CAD build for the part. Positions are in the model's coordinates, mm. A direction names the side the tool comes from. Round coordinates to 2 decimals unless told otherwise and drop trailing zeros. Write each loop counter-clockwise with the first axis right and the second up, starting at its lowest first coordinate (ties: lowest second). Pieces come first, ordered by that corner, then holes. Notation, with made-up numbers: (38.5, 65) - (77.5, 65) arc R23 cw to (77.5, 75) - close; hole circle Ø2 at (25, -0.75). An arc over 180 degrees is marked (long way). Answer in a Markdown table with one row per item.
```python
from build123d import *

# Parameters (mm, degrees)
BOSS_EXTRUDE1_DEPTH = 60
SKETCH4_W           = 10
SKETCH4_H           = 90
BOSS_EXTRUDE2_DEPTH = 45
SKETCH6_W           = 25
SKETCH6_H           = 10
BOSS_EXTRUDE3_DEPTH = 45
SKETCH8_W           = 10
SKETCH8_H           = 15
BOSS_EXTRUDE4_DEPTH = 90
CUT_EXTRUDE1_DEPTH  = 10
BOSS_EXTRUDE5_DEPTH = 20
CUT_EXTRUDE2_DEPTH  = 5
SKETCH12_W          = 10
SKETCH12_H          = 30.5
CUT_EXTRUDE3_DEPTH  = 5
BOSS_EXTRUDE6_DEPTH = 5


with BuildPart() as part:
    # Sketch1 → Boss-Extrude1 (new body)
    with BuildSketch(Plane(origin=(0, 0, 0), x_dir=(0, 0, -1), z_dir=(1, 0, 0))):
        Polygon((0, -10), (0, 90), (10, 90), (10, 0), (25, 0), (25, -10), align=None)
    extrude(amount=BOSS_EXTRUDE1_DEPTH)

    # Sketch4 → Boss-Extrude2 (add)
    with BuildSketch(Plane.ZY):
        with Locations((-5, 45)):
            Rectangle(SKETCH4_W, SKETCH4_H)
    extrude(amount=BOSS_EXTRUDE2_DEPTH)

    # Sketch6 → Boss-Extrude3 (add)
    with BuildSketch(Plane.ZY):
        with Locations((-12.5, -5)):
            Rectangle(SKETCH6_W, SKETCH6_H)
    extrude(amount=BOSS_EXTRUDE3_DEPTH)

    # Sketch8 → Boss-Extrude4 (add)
    with BuildSketch(Plane(origin=(0, 0, 0), x_dir=(1, 0, 0), z_dir=(0, 1, 0))):
        with Locations((-40, 17.5)):
            Rectangle(SKETCH8_W, SKETCH8_H)
    extrude(amount=BOSS_EXTRUDE4_DEPTH)

    # Sketch9 → Cut-Extrude1 (cut)
    with BuildSketch(Plane(origin=(0, 0, -10), x_dir=(-1, 0, 0), z_dir=(0, 0, -1))):
        with BuildLine():
            Line((-34.5, 40.5), (-60, 40.5))
            Line((-60, 40.5), (-60, 79.5))
            Line((-60, 79.5), (-34.5, 79.5))
            ThreePointArc((-34.5, 79.5), (-15, 60), (-34.5, 40.5))
        make_face()
    extrude(amount=-CUT_EXTRUDE1_DEPTH, mode=Mode.SUBTRACT)

    # Sketch10 → Boss-Extrude5 (add)
    with BuildSketch(Plane(origin=(0, 90, 0), x_dir=(1, 0, 0), z_dir=(0, 1, 0))):
        Polygon((60, 10), (-35, 10), (-35, 25), (-45, 25), (-45, 0), (60, 0), align=None)
    extrude(amount=BOSS_EXTRUDE5_DEPTH)

    # Sketch11 → Cut-Extrude2 (cut)
    with BuildSketch(Plane(origin=(60, 0, 0), x_dir=(0, 0, -1), z_dir=(1, 0, 0))):
        Polygon((10, 0), (10, 40.5), (0, 40.5), (0, -10), (25, -10), (25, 0), align=None)
    extrude(amount=-CUT_EXTRUDE2_DEPTH, mode=Mode.SUBTRACT)

    # Sketch12 → Cut-Extrude3 (cut)
    with BuildSketch(Plane(origin=(60, 0, 0), x_dir=(0, 0, -1), z_dir=(1, 0, 0))):
        with Locations((5, 94.75)):
            Rectangle(SKETCH12_W, SKETCH12_H)
    extrude(amount=-CUT_EXTRUDE3_DEPTH, mode=Mode.SUBTRACT)

    # Sketch13 → Boss-Extrude6 (add)
    with BuildSketch(Plane(origin=(0, 0, -25), x_dir=(-1, 0, 0), z_dir=(0, 0, -1))):
        Polygon((35, 0), (-55, 0), (-55, -10), (45, -10), (45, 110), (35, 110), align=None)
    extrude(amount=BOSS_EXTRUDE6_DEPTH)


solid = part.part
```
Q1. Drill centre lines: line 1 (Y direction, x = 42, z = -2); line 2 (Y direction, x = -3, z = -11.25); line 3 (X direction, y = 74, z = -19.75). Where is each one in solid material? Low to high.
Computed:
| item | result |
|---|---|
| line 1 | y = -10 to 40.5, 79.5 to 110 |
| line 2 | y = -10 to 0 |
| line 3 | x = -45 to -35 |
Q2. Saw through at D-D on x = 9.5. List the corners of the cut face in (y, z).
Computed:
| item | result |
|---|---|
| outline | (-10, -30) - (0, -30) - (0, -10) - (110, -10) - (110, 0) - (-10, 0) - close |
Q3. Saw through at A-A on x = 40.5. List the corners of the cut face in (y, z).
Computed:
| item | result |
|---|---|
| outline | (-10, -30) - (0, -30) - (0, -10) - (40.5, -10) - (40.5, 0) - (-10, 0) - close; (79.5, -10) - (110, -10) - (110, 0) - (79.5, 0) - close |
Q4. Flat gauge pin, fed straight in: pin 1 (1 mm diameter, centred on x = -19, z = -13, fed in from +Y). Where does the tip first touch, or does it go through?
Computed:
| item | result |
|---|---|
| pin 1 | stops at y = 0 |
Q5. Saw through at B-B on z = -2.75. List the corners of the cut face in (x, y), then the cut area to 3 significant figures.
Computed:
| item | result |
|---|---|
| outline | (-45, -10) - (55, -10) - (55, 40.5) - (34.5, 40.5) arc R19.5 cw to (34.5, 79.5) - (55, 79.5) - (55, 110) - (-45, 110) - close |
| area | 10,600 mm2 |
Q6. 3-axis set-ups, long thin cutter, end or side, ignore diameter. For faces 1 (the flat face through (-7, 110, -8)), 2 (the flat face through (45, 40.5, -5)), 3 (the flat face through (9, 0, -20)): which of +Z, -Z, +X, -X, +Y, -Y reach the whole face in a straight line?
Computed:
| item | result |
|---|---|
| face 1 | +Z, -Z, +X, -X, +Y |
| face 2 | +Z, -Z, +X |
| face 3 | -Z, +X, +Y |
Q7. Pull direction Y, two halves, no side cores. Call faces 4 (the flat face through (45, 79.5, -5)), 5 (the flat face through (6, -10, -15)), 6 (the flat face through (4, 49, 0)): released by +Y, released by -Y, zero draft, split by the parting line, or undercut.
Computed:
| item | result |
|---|---|
| face 4 | undercut |
| face 5 | released by -Y |
| face 6 | zero draft |
Q8. Saw through at C-C on y = 93. List the corners of the cut face in (x, z), then the cut area to 3 significant figures.
Computed:
| item | result |
|---|---|
| outline | (-45, -30) - (-35, -30) - (-35, -10) - (55, -10) - (55, 0) - (-45, 0) - close |
| area | 1,200 mm2 |
